```python
from build123d import *

# Parameters (mm, degrees)
SKETCH2_R           = 1.75
BOSS_EXTRUDE1_DEPTH = 3
FILLET1_R           = 4.16054


with BuildPart() as part:
    # Sketch2 → Boss-Extrude1 (new body)
    with BuildSketch(Plane.XY):
        with BuildLine():
            Line((18.479229397, -39.61885681), (20.435570278, -43.813186973))
            ThreePointArc((20.435570278, -43.813186973), (45.250304059, 8.388683548), (0, 44.35))
            Line((0, 44.35), (0, 52.75))
            ThreePointArc((0, 52.75), (52.298716437, 6.88525664), (13.652704629, -50.952587337))
            Line((13.652704629, -50.952587337), (11.314672737, -42.226933525))
            Line((11.314672737, -42.226933525), (18.479229397, -39.61885681))
        make_face()
        with Locations((16.470452213, -45.245405335)):
            Circle(SKETCH2_R, mode=Mode.SUBTRACT)
    extrude(amount=BOSS_EXTRUDE1_DEPTH)

    # Fillet1
    fillet1_edges = [part.edges().sort_by_distance(p)[0] for p in [
        (18.479229397, -39.61885681, 1.5),
        (11.314672737, -42.226933525, 1.5),
    ]]
    fillet(fillet1_edges, radius=FILLET1_R - 0.0001)  # a hair under: the kernel refuses the full size

    # Mirror1: part across plane


with BuildPart() as part_1:
    add(part.part)
    add(part.part.mirror(Plane(origin=(0, 52.75, 3), x_dir=(0, 0, 1), z_dir=(1, 0, 0))))


solid = part_1.part
```
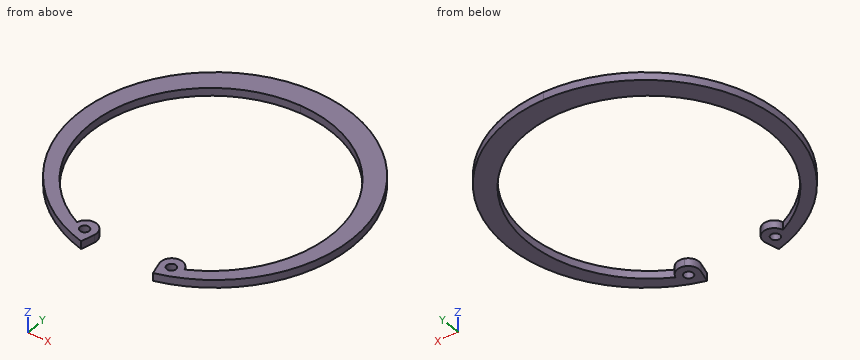
Verification items for the finished model (mm, model axes). Coordinates: 2 decimals unless noted, no trailing zeros. Write each loop counter-clockwise with the first axis right and the second up, starting at its lowest first coordinate (ties: lowest second). Pieces come first, ordered by that corner, then holes. Notation, with made-up numbers: M 37.25,47 L 67.25,47 A34 ccw 67.25,86 Z; hole C 77.25,60.5 d8. An arc over 180 degrees is marked long. Answer as a JSON object with one key per item and string values. Group by question number.
(1) Gauge pin test, flat ends, axial feed: pin 1 (1.5 mm diameter, centred on y = -28, z = 2, fed in from -X); pin 2 (3 mm diameter, centred on x = -16.47, y = -45.25, fed in from +Z). Record the tip position at first contact, or that the pin passes through.
(2) Material ranges on line 1 (X direction, y = -44.5, z = 2.3); line 2 (Y direction, x = 37.5, z = 0.3); line 3 (Y direction, x = -38, z = 2.1), recorded low to high.
(3) Cross-section at A-A, the plane y = -36. Record the cut outline in (x, z).
(4) Cross-section at C-C, the plane z = 0.75. State how many separate pieces and enclosed holes the cut face has, and give its area (3 significant figures).
(5) Cross-section at B-B, the plane x = -39. Record the cut outline in (y, z), and give its area (3 significant figures).
Reply:
{
 "1": {"pin 1": "x = -45.17", "pin 2": "through"},
 "2": {"line 1": "-28.33 to -18.05, -14.89 to -12.17, 12.17 to 14.89, 18.05 to 28.33", "line 2": "-37.1 to -29.51, 25.31 to 37.1", "line 3": "-36.59 to -28.81, 24.61 to 36.59"},
 "3": {"outline": "M -38.56,0 L -31.76,0 L -31.76,3 L -38.56,3 Z; M 31.76,0 L 38.56,0 L 38.56,3 L 31.76,3 Z"},
 "4": {"separate pieces": "1", "enclosed holes": "2", "area": "1,900 mm²"},
 "5": {"outline": "M -35.52,0 L -27.33,0 L -27.33,3 L -35.52,3 Z; M 23.13,0 L 35.52,0 L 35.52,3 L 23.13,3 Z", "area": "61.7 mm²"}
}
